from build123d import *

# Parameters (mm, degrees)
F0_R     = 7.1
F1_DEPTH = 1
F2_DEPTH = 6
F3_R     = 0.5
F6_DEPTH = 4.3


with BuildPart() as f1:
    # F0 (on Top) → F1 (new body)
    with BuildSketch(Plane.XY):
        Circle(F0_R)
        with BuildLine():
            ThreePointArc((-1.4720513892, -4.8829360745), (-3.0415898733, 4.0937429136), (5.1, 0))
            ThreePointArc((5.1, 0), (4.0937429136, -3.0415898733), (1.4720513892, -4.8829360745))
            ThreePointArc((1.4720513892, -4.8829360745), (1.3862386511, -4.9079876123), (1.3, -4.9315312024))
            ThreePointArc((1.3, -4.9315312024), (0, -5.1), (-1.3, -4.9315312024))
            ThreePointArc((-1.3, -4.9315312024), (-1.3862386511, -4.9079876123), (-1.4720513892, -4.8829360745))
        make_face(mode=Mode.SUBTRACT)
    extrude(amount=F1_DEPTH)

    # F0 (on Top) → F2 (join)
    with BuildSketch(Plane.XY):
        with BuildLine():
            ThreePointArc((1.4720513892, -4.8829360745), (4.0937429136, -3.0415898733), (5.1, 0))
            ThreePointArc((5.1, 0), (-3.0415898733, 4.0937429136), (-1.4720513892, -4.8829360745))
            Line((-1.4720513892, -4.8829360745), (-1.3, -1.6))
            Line((-1.3, -1.6), (1.3, -1.6))
            Line((1.3, -1.6), (1.4720513892, -4.8829360745))
        make_face()
    extrude(amount=F2_DEPTH)

    # F3
    f3_edges = [f1.edges().sort_by_distance(p)[0] for p in [
        (-1.3, -1.6, 3),
        (1.3, -1.6, 3),
    ]]
    fillet(f3_edges, radius=F3_R)

    # F5 (on offset) → F6 (cut)
    with BuildSketch(Plane.XY.offset(6)):
        Polygon((2.3, 0.8), (-2.3, 0.8), (-2.3, -2.7), (-1.3, -2.7), (1.3, -2.7), (2.3, -2.7), align=None)
    extrude(amount=-F6_DEPTH, mode=Mode.SUBTRACT)


solid = f1.part
For this review, take the finished solid that the model builds, in its own axes (mm). A direction names the side the tool comes from. Coordinates: 2 decimals unless noted, no trailing zeros. Order: outer loops, then holes, each group sorted by start corner. A loop starts at its lowest first (then second) coordinate and runs counter-clockwise, first axis right, second up. Notation, with made-up numbers: (74.5, 79) - (127.5, 79) arc R35 cw to (127.5, 117) - close; hole circle Ø2 at (42, -38). An arc over 180 degrees is marked (long way). Answer as CSV lines item,"result". Start each with the question number.
1) Add section C-C (z = 1.35). State the section outline as (x, y) points, then the cut area to 3 significant figures.
2) Draft analysis for pull direction Y (two halves, no side actions). For faces 4 (the cylindrical face through (-0.92, 7.04, 0.49)), 5 (the flat face through (0, 1, 6)), 6 (the flat face through (0, -1.6, 1)), state which applies: +Y half, -Y half, draft (parallel to the pull), parting line (faces both ways), or undercut.
3) Add section D-D (y = -4). State the section outline as (x, z) points.
4) Insertion check: P1, Ø1.8, axis at y = -1.5, z = 3.5, coming from the +X side; P2, Ø0.5, axis at x = -0.5, z = 1, coming from the -Y side; P3, Ø1, axis at x = 1, y = -1, coming from the +Z side; P4, Ø3, axis at x = 5, y = -4, coming from the -Z side. Each pin has a flat end and moves straight along its axis. Give the tip position at first contact, or say it passes through.
5) Add section A-A (x = 0). State the section outline as (y, z) points.
6) To check wall thickness, follow line 1 along X through (y, z) = (0, 1.5); line 2 along Z through (x, y) = (-2.25, -5.5); line 3 along X through (y, z) = (-0.75, 4.15). State the ranges of each line that lie inside material, in increasing order. Write a range as [from, to].
7) Machinability: for faces 1 (the flat face through (1.414, -3.771, 2.958)), 2 (the flat face through (0, 0.8, 4)), 3 (the flat face through (0, 0, 0)), which of the approach directions +Z, -Z, +X, -X, +Y, -Y give a long, thin tool a straight path to every point of the face, cutting with its end or side? Answer none if there is none.
8) Add section B-B (z = 0.4). State the section outline as (x, y) points, then the cut area to 3 significant figures.
Result:
1,outline,"(-1.47, -4.88) - (-1.32, -2.07) arc R0.5 cw to (-0.83, -1.6) - (0.83, -1.6) arc R0.5 cw to (1.32, -2.07) - (1.47, -4.88) arc R5.1 ccw (long way) to start"
1,area,"72.3 mm^2"
2,face 4,"parting line"
2,face 5,"draft"
2,face 6,"undercut"
3,outline,"(-5.87, 0) - (-1.43, 0) - (-1.43, 6) - (-3.16, 6) - (-3.16, 1) - (-5.87, 1) - close; (1.43, 0) - (5.87, 0) - (5.87, 1) - (3.16, 1) - (3.16, 6) - (1.43, 6) - close"
4,P1,"x = 5.06"
4,P2,"y = -7.1"
4,P3,"z = 1.7"
4,P4,"z = 0"
5,outline,"(-7.1, 0) - (-5.1, 0) - (-5.1, 1) - (-7.1, 1) - close; (-1.6, 0) - (7.1, 0) - (7.1, 1) - (5.1, 1) - (5.1, 6) - (0.8, 6) - (0.8, 1.7) - (-1.6, 1.7) - close"
6,line 1,"[-5.1, 5.1]"
6,line 2,"[0, 1]"
6,line 3,"[-5.04, -2.3], [2.3, 5.04]"
7,face 1,"+Z, -Z"
7,face 2,"+Z"
7,face 3,"-Z, +X, -X, +Y, -Y"
8,outline,"circle Ø14.2 at (0, 0); hole (-1.47, -4.88) arc R5.1 ccw to (1.47, -4.88) - (1.32, -2.07) arc R0.5 ccw to (0.83, -1.6) - (-0.83, -1.6) arc R0.5 ccw to (-1.32, -2.07) - close"
8,area,"149 mm^2"
